The model under review builds one solid part; all positions refer to its coordinate system, in mm. A direction names the side the tool comes from. Round coordinates to 2 decimals unless told otherwise and drop trailing zeros. Write each loop counter-clockwise with the first axis right and the second up, starting at its lowest first coordinate (ties: lowest second). Pieces come first, ordered by that corner, then holes.
Item 1: Draft analysis for pull direction Y (two halves, no side actions). For faces 4 (the face through (-10.652, -31.047, 3.005)), 5 (the face through (0, -26, 3)), 6 (the face through (-25.22, -1.88, 3.01)), state which applies: +Y half, -Y half, draft (parallel to the pull), parting line (faces both ways), or undercut.
Item 2: Add section C-C (x = -6). Give the boundary of the cut face in (y, z).
Item 3: Add section A-A (x = -34.5). Give the boundary of the cut face in (y, z) (3 decimals).
Item 4: Add section D-D (z = 3.75). Give the boundary of the cut face in (x, y) (3 decimals), plus the area to 3 significant figures.
Item 5: Clearance check with flat-ended pins moving along their axes: pin 1 Ø1.8 at (y, z) = (-42.5, 3.5) entering from -X; pin 2 Ø1.7 at (x, z) = (-35.5, 3.5) entering from -Y; pin 3 Ø3 at (x, z) = (-25.5, 4) entering from -Y. State where each tip first meets the part, or that it passes through.
Item 6: Machinability: for faces 1 (the face through (-35, -24.003, 3)), 2 (the face through (-19, -35, 0)), 3 (the face through (-7.857, -19.22, 3.005)), which of the approach directions +Z, -Z, +X, -X, +Y, -Y give a long, thin tool a straight path to every point of the face, cutting with its end or side? Answer none if there is none.
Item 7: To check wall thickness, follow L1, parallel to Y at x = -35.5, z = 4.5 (3 decimals); L2, parallel to X at y = -14, z = 5; L3, parallel to Y at x = -10.5, z = 0.5. State the ranges of each line that lie inside material, in increasing order.
Item 8: Add section B-B (y = -7). Give the boundary of the cut face in (x, z).
```python
from build123d import *

# Parameters (mm, degrees)
SKETCH1_R           = 3.048
BOSS_EXTRUDE1_DEPTH = 6.096
CUT_EXTRUDE1_DEPTH  = 8.636
SKETCH4_W           = 5.715
SKETCH4_H           = 7.239
CUT_EXTRUDE2_DEPTH  = 81.243500547
SKETCH5_R           = 1.524
CUT_EXTRUDE4_DEPTH  = 6.096


with BuildPart() as part:
    # Sketch1 → Boss-Extrude1 (new body)
    with BuildSketch(Plane.XY):
        Polygon((0, 0), (-38.1, 0), (-38.1, -8.255), (-32.131, -8.255), (-32.131, -15.748), (-38.1, -15.748), (-38.1, -24.003), (-32.131, -24.003), (-32.131, -31.496), (-38.1, -31.496), (-38.1, -39.751), (-32.131, -39.751), (-32.131, -47.244), (-38.1, -47.244), (-38.1, -70.358), (0, -50.8), align=None)
        with Locations(Location((-8.382, -8.382, 0), (0, 0, 180))):
            Circle(SKETCH1_R, mode=Mode.SUBTRACT)
    extrude(amount=BOSS_EXTRUDE1_DEPTH)

    # Sketch2 → Cut-Extrude1 (cut)
    with BuildSketch(Plane(origin=(0, 0, 0), x_dir=(-1, 0, 0), z_dir=(0, 0, -1))):
        Polygon((38.1, 0), (12.7, 0), (38.1, -3.81), align=None)
    extrude(amount=-CUT_EXTRUDE1_DEPTH, mode=Mode.SUBTRACT)

    # Sketch4 → Cut-Extrude2 (cut, through all)
    with BuildSketch(Plane.XY.offset(6.096)):
        with Locations((-35.2425, -58.8645)):
            Rectangle(SKETCH4_W, SKETCH4_H)
    extrude(amount=-CUT_EXTRUDE2_DEPTH, mode=Mode.SUBTRACT)

    # Sketch5 → Cut-Extrude4 (cut)
    with BuildSketch(Plane(origin=(0, 0, 0), x_dir=(-1, 0, 0), z_dir=(0, 0, -1))):
        with Locations((10.982204311, -29.558964691)):
            Circle(SKETCH5_R)
        Polygon((7.629906021, -17.367131003), (11.285453498, -16.918286212), (11.73429829, -20.573833688), (8.078750813, -21.02267848), align=None)
    extrude(amount=-CUT_EXTRUDE4_DEPTH, mode=Mode.SUBTRACT)


solid = part.part
```
Numbers:
1. face 4: undercut
1. face 5: draft
1. face 6: +Y half
2. outline: (-53.88, 0) - (-10.28, 0) - (-10.28, 6.1) - (-53.88, 6.1) - close; (-6.48, 0) - (0, 0) - (0, 6.1) - (-6.48, 6.1) - close
3. outline: (-68.51, 0) - (-62.484, 0) - (-62.484, 6.096) - (-68.51, 6.096) - close; (-55.245, 0) - (-47.244, 0) - (-47.244, 6.096) - (-55.245, 6.096) - close; (-39.751, 0) - (-31.496, 0) - (-31.496, 6.096) - (-39.751, 6.096) - close; (-24.003, 0) - (-15.748, 0) - (-15.748, 6.096) - (-24.003, 6.096) - close; (-8.255, 0) - (-3.27, 0) - (-3.27, 6.096) - (-8.255, 6.096) - close
4. outline: (-38.1, -70.358) - (0, -50.8) - (0, 0) - (-12.7, 0) - (-38.1, -3.81) - (-38.1, -8.255) - (-32.131, -8.255) - (-32.131, -15.748) - (-38.1, -15.748) - (-38.1, -24.003) - (-32.131, -24.003) - (-32.131, -31.496) - (-38.1, -31.496) - (-38.1, -39.751) - (-32.131, -39.751) - (-32.131, -47.244) - (-38.1, -47.244) - (-38.1, -55.245) - (-32.385, -55.245) - (-32.385, -62.484) - (-38.1, -62.484) - close; hole circle Ø3.048 at (-10.982, -29.559); hole (-11.734, -20.574) - (-8.079, -21.023) - (-7.63, -17.367) - (-11.285, -16.918) - close; hole circle Ø6.096 at (-8.382, -8.382)
4. area: 2,030 mm2
5. pin 1: stops at x = -32.13
5. pin 2: stops at y = -69.46
5. pin 3: stops at y = -64.66
6. face 1: +Z, -Z, -X
6. face 2: -Z, +X, -X, +Y, -Y
6. face 3: +Z, -Z
7. L1: y = -69.023 to -62.484, -55.245 to -47.244, -39.751 to -31.496, -24.003 to -15.748, -8.255 to -3.42
7. L2: x = -32.13 to 0
7. L3: y = -56.19 to -31, -28.11 to -20.73, -17.01 to -10.57, -6.19 to 0
8. outline: (-38.1, 0) - (-11.1, 0) - (-11.1, 6.1) - (-38.1, 6.1) - close; (-5.67, 0) - (0, 0) - (0, 6.1) - (-5.67, 6.1) - close
